```python
from build123d import *

# Parameters (mm, degrees)
BOSS_EXTRUDE3_DEPTH = 50
CUT_EXTRUDE2_DEPTH  = 120.036992567
SKETCH12_W          = 16.875844183
SKETCH12_H          = 25.353739704
CUT_EXTRUDE3_DEPTH  = 114.190623836


with BuildPart() as part:
    # Sketch7 → Boss-Extrude3 (new body)
    with BuildSketch(Plane(origin=(0, 0, 0), x_dir=(0, 0, -1), z_dir=(1, 0, 0))):
        with BuildLine():
            ThreePointArc((55.561833342, 64.861882699), (27.780916671, 92.64279937), (0, 64.861882699))
            Line((0, 64.861882699), (55.561833342, 64.861882699))
        make_face()
        with BuildLine():
            Line((55.561833342, 64.861882699), (0, 64.861882699))
            ThreePointArc((0, 64.861882699), (27.780916671, 37.080966028), (55.561833342, 64.861882699))
        make_face()
        with BuildLine():
            Line((0, 64.861882699), (0, 0))
            Line((0, 0), (55.561833342, 0))
            Line((55.561833342, 0), (55.561833342, 64.861882699))
            ThreePointArc((55.561833342, 64.861882699), (27.780916671, 37.080966028), (0, 64.861882699))
        make_face()
    extrude(amount=BOSS_EXTRUDE3_DEPTH)

    # Sketch8 → Cut-Extrude2 (cut, through all)
    with BuildSketch(Plane(origin=(50, 0, 0), x_dir=(0, 0, -1), z_dir=(1, 0, 0))):
        with BuildLine():
            ThreePointArc((41.196796873, 67.582158988), (28.519927021, 80.25902884), (15.843057169, 67.582158988))
            Line((15.843057169, 67.582158988), (41.196796873, 67.582158988))
        make_face()
        with BuildLine():
            Line((41.196796873, 67.582158988), (15.843057169, 67.582158988))
            ThreePointArc((15.843057169, 67.582158988), (28.519927021, 54.905289136), (41.196796873, 67.582158988))
        make_face()
        with BuildLine():
            ThreePointArc((41.196796873, 67.582158988), (28.519927021, 54.905289136), (15.843057169, 67.582158988))
            Line((15.843057169, 67.582158988), (15.843057169, 0))
            Line((15.843057169, 0), (41.196796873, 0))
            Line((41.196796873, 0), (41.196796873, 67.582158988))
        make_face()
    extrude(amount=-CUT_EXTRUDE2_DEPTH, mode=Mode.SUBTRACT)

    # Sketch12 → Cut-Extrude3 (cut, through all)
    with BuildSketch(Plane(origin=(0, 85, 0), x_dir=(1, 0, 0), z_dir=(0, 1, 0))):
        with Locations((25.070624904, 28.519927021)):
            Rectangle(SKETCH12_W, SKETCH12_H)
    extrude(amount=CUT_EXTRUDE3_DEPTH, mode=Mode.SUBTRACT)


solid = part.part
```
Part model, mm, in its own coordinate system. A direction names the side the tool comes from. Round coordinates to 2 decimals unless told otherwise and drop trailing zeros. Loops run counter-clockwise (first coordinate to the right, second up) from the corner with the lowest first, then second, coordinate; pieces in that order, holes last.
Item 1: Mould opens along X. For faces 1 (the face through (50, 47, -15)), 2 (the face through (25, 0, -8)), 3 (the face through (25, 87, -15.843)) say: +X half, -X half, draft (parallel to the pull), parting line (faces both ways), or undercut.
Item 2: Cut at A-A, the plane y = 30. Give the cut face in (x, z).
Item 3: Cut at B-B, the plane x = 35. Give the cut face in (y, z), then the cut area to 3 significant figures.
Item 4: Drop flat-ended pins along their axis: P1, Ø12, axis at x = 33.5, y = 79, coming from the +Z side; P2, Ø2.5, axis at x = 27.5, y = 86.5, coming from the -Z side; P3, Ø10, axis at x = 37.5, z = -11, coming from the +Y side. Give the stop position or say it passes through.
Item 5: Cut at D-D, the plane y = 87. Give the cut face in (x, z), then the cut area to 3 significant figures.
Item 6: Drill centre lines: line 1 (Z direction, x = 24, y = 52.5); line 2 (Z direction, x = 36, y = 77); line 3 (Y direction, x = 32, z = -28). Where is each one in solid material? Low to high.
Item 7: Cut at C-C, the plane z = -17. Give the cut face in (x, y).
Item 8: 3-axis set-ups, long thin cutter, end or side, ignore diameter. For faces 4 (the face through (25, 33, -41.197)), 5 (the face through (25, 33, 0)), 6 (the face through (33.509, 89, -28)): which of +Z, -Z, +X, -X, +Y, -Y reach the whole face in a straight line?
A:
1. face 1: +X half
1. face 2: draft
1. face 3: undercut
2. outline: (0, -55.56) - (50, -55.56) - (50, -41.2) - (0, -41.2) - close; (0, -15.84) - (50, -15.84) - (50, 0) - (0, 0) - close
3. outline: (0, -55.56) - (64.86, -55.56) arc R27.78 ccw to (64.86, 0) - (0, 0) - (0, -15.84) - (67.58, -15.84) arc R12.68 cw to (67.58, -41.2) - (0, -41.2) - close
3. area: 2,850 mm2
4. P1: stops at z = -1.22
4. P2: stops at z = -46.65
4. P3: stops at y = 90.02
5. outline: (0, -44.56) - (50, -44.56) - (50, -11) - (0, -11) - close; hole (16.63, -41.2) - (33.51, -41.2) - (33.51, -15.84) - (16.63, -15.84) - close
5. area: 1,250 mm2
6. line 1: z = -55.56 to -41.2, -15.84 to 0
6. line 2: z = -52.77 to -37.01, -20.03 to -2.79
6. line 3: y = 80.25 to 85
7. outline: (0, 72.87) - (50, 72.87) - (50, 90.47) - (33.51, 90.47) - (33.51, 85) - (16.63, 85) - (16.63, 90.47) - (0, 90.47) - close
8. face 4: +X, -X, -Y
8. face 5: +Z, +X, -X, +Y, -Y
8. face 6: +Y
